Source: three-view drawing plus pictorial views. Frame: mm from the lowest corner of the part. Coordinates: 2 decimals unless noted, no trailing zeros. Order: outer loops, then holes, each group sorted by start corner. A loop starts at its lowest first (then second) coordinate and runs counter-clockwise, first axis right, second up. Notation, with made-up numbers: (-26, 26) - (12, 26) arc R5 ccw to (12, 34) - close; hole circle Ø1 at (44, -25.5). An arc over 180 degrees is marked (long way). One line per question, with ' | ' between items.
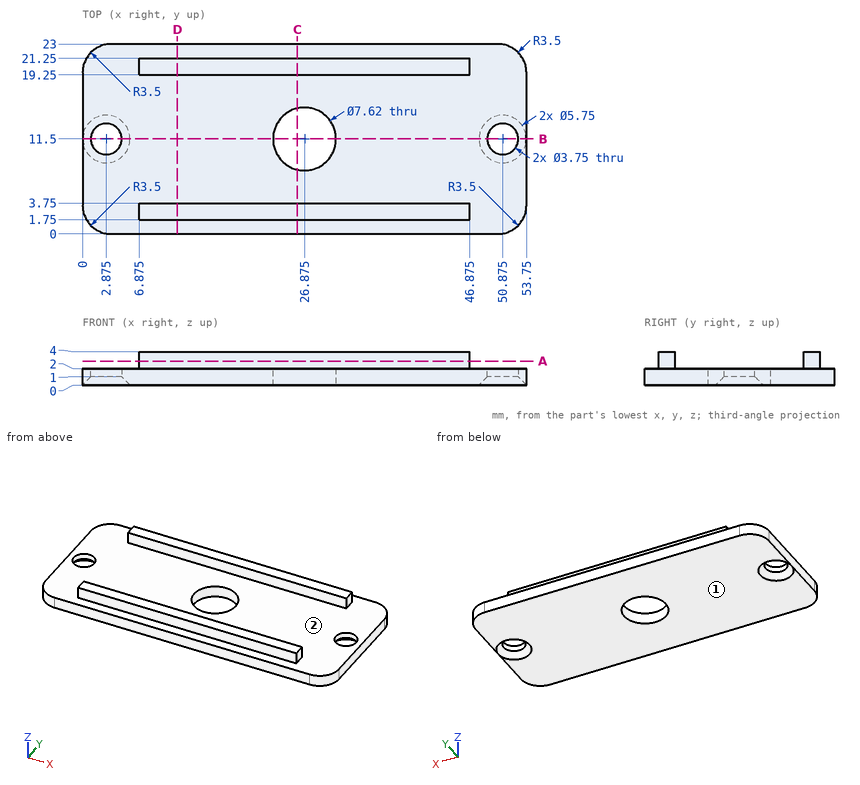
(1) Cut plane B-B (y = 11.5). State how many separate pieces and enclosed holes the cut face has, and give its area (3 significant figures).
Taken from the geometry:
separate pieces: 4 | enclosed holes: 0 | area: 75.3 mm²
(2) Pull-direction query (Y, two-part tool) for the marked faces 1 and 2; classes: pulls with the +Y half, pulls with the -Y half, needs draft (parallel to the pull), parting line crosses it, or undercut.
Taken from the geometry:
face 1: needs draft | face 2: undercut
(3) Material intervals for L1, parallel to Y at x = 25, z = 3.5; L2, parallel to Z at x = 42, y = 17.5; L3, parallel to X at y = 21, z = 2.5 (3 decimals), sorted ascending. Write a range as from..to.
Taken from the geometry:
L1: y = 1.75..3.75, 19.25..21.25 | L2: z = 0..2 | L3: x = 6.875..46.875
(4) Cut plane A-A (z = 2.9). Return the cut outline in (x, y) (3 decimals).
Taken from the geometry:
outline: (6.875, 1.75) - (46.875, 1.75) - (46.875, 3.75) - (6.875, 3.75) - close; (6.875, 19.25) - (46.875, 19.25) - (46.875, 21.25) - (6.875, 21.25) - close
(5) Pin query (flat end, axial travel): P1, Ø0.6, axis at x = 18.5, z = 2.5, coming from the +Y side; P2, Ø0.6, axis at x = 36, z = 3, coming from the -Y side; P3, Ø4.5, axis at x = 26.875, y = 11.5, coming from the +Z side; P4, Ø0.6, axis at y = 20, z = 2.5, coming from the +X side (3 decimals). Return the tip coordinate at first contact, or that it passes through.
Taken from the geometry:
P1: stops at y = 21.25 | P2: stops at y = 1.75 | P3: passes through | P4: stops at x = 46.875
(6) Cut plane C-C (x = 26). Return the cut outline in (y, z).
Taken from the geometry:
outline: (0, 0) - (7.79, 0) - (7.79, 2) - (3.75, 2) - (3.75, 4) - (1.75, 4) - (1.75, 2) - (0, 2) - close; (15.21, 0) - (23, 0) - (23, 2) - (21.25, 2) - (21.25, 4) - (19.25, 4) - (19.25, 2) - (15.21, 2) - close
(7) Cut plane D-D (x = 11.5). Return the cut outline in (y, z).
Taken from the geometry:
outline: (0, 0) - (23, 0) - (23, 2) - (21.25, 2) - (21.25, 4) - (19.25, 4) - (19.25, 2) - (3.75, 2) - (3.75, 4) - (1.75, 4) - (1.75, 2) - (0, 2) - close
